Build history of the part. All positions in model axes, mm. Face numbers are marked on the shaded views. A direction names the side the tool comes from. Round coordinates to 2 decimals unless told otherwise and drop trailing zeros. Loops run counter-clockwise (first coordinate to the right, second up) from the corner with the lowest first, then second, coordinate; pieces in that order, holes last. Notation, with made-up numbers: (-17, 30.5) -> (8, 30.5) arc R35 cw to (8, 66.5) -> close; hole circle Ø10 at (-12.75, -9.75). An arc over 180 degrees is marked (long way). Put each result on its own line as item: value. Start each with the question number.
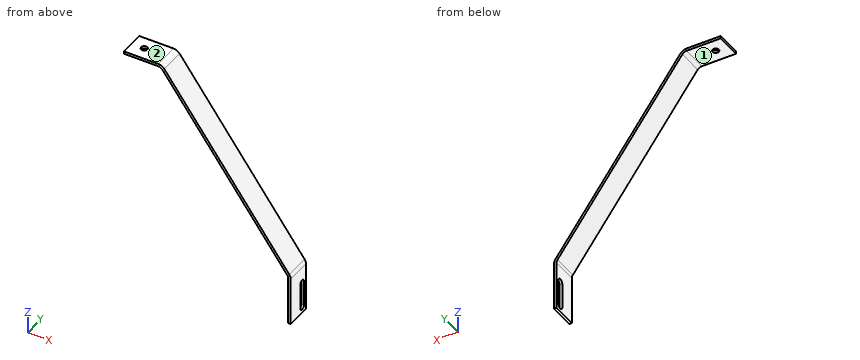
```python
from build123d import *

# Parameters (mm, degrees)
BOSS_EXTRUDE1_DEPTH  = 20
CONVERT_SOLID2_DEPTH = 20
SKETCH8_R            = 2.5
CUT_EXTRUDE1_DEPTH   = 20
CUT_EXTRUDE2_DEPTH   = 10


# Read off the part's stored shape, not the designer's step: Convert-Solid2
with BuildPart() as part:
    # Sketch1 → Boss-Extrude1 (new body)
    with BuildSketch(Plane(origin=(0, 0, 0), x_dir=(1, 0, 0), z_dir=(0, 1, 0))):
        Polygon((0, 0), (30, 0), (131.25, 140), (131.25, 180), (126.25, 180), (126.25, 141.618570234), (27.445498313, 5), (0, 5), align=None)
    extrude(amount=BOSS_EXTRUDE1_DEPTH)

    # Convert-Solid2 outline → Convert-Solid2 (cut)
    with BuildSketch(Plane(origin=(0, 0, 0), x_dir=(1, 0, 0), z_dir=(0, 1, 0))):
        with BuildLine():
            Line((30, 0), (31.796383005, 2.483887612))
            ThreePointArc((31.796383005, 2.483887612), (29.664371379, 0.656935602), (26.934597975, 0))
            Line((26.934597975, 0), (30, 0))
        make_face()
        with BuildLine():
            ThreePointArc((131.25, 141.942284281), (130.958358353, 140.094408498), (130.11178503, 138.426171893))
            Line((130.11178503, 138.426171893), (131.25, 140))
            Line((131.25, 140), (131.25, 141.942284281))
        make_face()
        with BuildLine():
            Line((0, 5), (0, 2))
            Line((0, 2), (26.934597975, 2))
            ThreePointArc((26.934597975, 2), (28.754446911, 2.437957068), (30.175787995, 3.655925075))
            Line((30.175787995, 3.655925075), (128.49119002, 139.598209356))
            ThreePointArc((128.49119002, 139.598209356), (129.055572236, 140.710367092), (129.25, 141.942284281))
            Line((129.25, 141.942284281), (129.25, 180))
            Line((129.25, 180), (126.25, 180))
            Line((126.25, 180), (126.25, 141.618570234))
            Line((126.25, 141.618570234), (27.445498313, 5))
            Line((27.445498313, 5), (0, 5))
        make_face()
    extrude(amount=CONVERT_SOLID2_DEPTH, mode=Mode.SUBTRACT)

    # Sketch8 → Cut-Extrude1 (cut)
    with BuildSketch(Plane.XY):
        with Locations((10, 10)):
            Circle(SKETCH8_R)
    extrude(amount=-CUT_EXTRUDE1_DEPTH, mode=Mode.SUBTRACT)

    # Sketch9 → Cut-Extrude2 (cut)
    with BuildSketch(Plane(origin=(131.25, 0, -320.372504423), x_dir=(0, 0, 1), z_dir=(-1, 0, 0))):
        with BuildLine():
            Line((145.372504423, 17.5), (165.372504423, 17.5))
            ThreePointArc((165.372504423, 17.5), (167.872504423, 15), (165.372504423, 12.5))
            Line((165.372504423, 12.5), (145.372504423, 12.5))
            ThreePointArc((145.372504423, 12.5), (142.872504423, 15), (145.372504423, 17.5))
        make_face()
    extrude(amount=CUT_EXTRUDE2_DEPTH, mode=Mode.SUBTRACT)


solid = part.part
```
Item 1: Cut at B-B on x = 10. Write the cut outline in (y, z), then the cut area to 3 significant figures.
Item 2: 3-axis set-ups, long thin cutter, end or side, ignore diameter. For the marked faces 1 and 2: which of +Z, -Z, +X, -X, +Y, -Y reach the whole face in a straight line?
Item 3: Drop flat-ended pins along their axis: pin 1 (6.5 mm diameter, centred on x = 10, y = 10, fed in from -Z); pin 2 (6 mm diameter, centred on y = 4.5, z = -125, fed in from -X); pin 3 (10 mm diameter, centred on x = 45.5, y = 12.5, fed in from +Z); pin 4 (2 mm diameter, centred on x = 130, z = -162.5, fed in from -Y). Give the stop position or say it passes through.
Item 4: Cut at C-C on z = -75. Write the cut outline in (x, y), then the cut area to 3 significant figures.
Item 5: Cut at D-D on x = 63. Write the cut outline in (y, z), then the cut area to 3 significant figures.
Item 6: Cut at A-A on y = 15. Write the cut outline in (x, z), then the cut area to 3 significant figures.
Item 7: Wall check: line 1 (Y direction, x = 10, z = -1); line 2 (X direction, y = 13.25, z = -145.5); line 3 (Z direction, x = 18, y = 6). Give the ranges that are in metal, low to high. Write a range as from..to.
Ans:
1. outline: (0, -2) -> (7.5, -2) -> (7.5, 0) -> (0, 0) -> close; (12.5, -2) -> (20, -2) -> (20, 0) -> (12.5, 0) -> close
1. area: 30.0 mm2
2. face 1: -Z, -X, +Y, -Y
2. face 2: +Z, +X, -X, +Y, -Y
3. pin 1: stops at z = -2
3. pin 2: stops at x = 115.76
3. pin 3: stops at z = -14.52
3. pin 4: stops at y = 0
4. outline: (81.77, 0) -> (84.24, 0) -> (84.24, 20) -> (81.77, 20) -> close
4. area: 49.4 mm2
5. outline: (0, -49.04) -> (20, -49.04) -> (20, -45.63) -> (0, -45.63) -> close
5. area: 68.3 mm2
6. outline: (0, -2) -> (26.93, -2) arc R4 cw to (30.18, -3.66) -> (128.49, -139.6) arc R4 cw to (129.25, -141.94) -> (129.25, -152.5) -> (131.25, -152.5) -> (131.25, -141.94) arc R6 ccw to (130.11, -138.43) -> (31.8, -2.48) arc R6 ccw to (26.93, 0) -> (0, 0) -> close; (129.25, -180) -> (131.25, -180) -> (131.25, -177.5) -> (129.25, -177.5) -> close
6. area: 431 mm2
7. line 1: y = 0..7.5, 12.5..20
7. line 2: x = 129.25..131.25
7. line 3: z = -2..0
